Input: part model. Units: mm. Frame: model coordinates. Face numbers are marked on the shaded views. A direction names the side the tool comes from. Coordinates: 2 decimals unless noted, no trailing zeros. Write each loop counter-clockwise with the first axis right and the second up, starting at its lowest first coordinate (ties: lowest second). Pieces come first, ordered by that corner, then holes. Notation, with made-up numbers: (55.25, 3.25) - (70.25, 3.25) arc R20 cw to (70.25, 27.25) - close; hole circle Ø6 at (11, -13). An arc over 180 degrees is marked (long way). Put each result on its own line as item: value. Start each with the question number.
1. Cut plane B-B, the plane z = 0. Return loops of the section in (x, y).
2. Line query: line 1 (Y direction, x = -5.25, z = -2.5); line 2 (X direction, y = 45, z = 3.5); line 3 (X direction, y = 14, z = 2.5). Output: solid intervals per line, ascending.
3. Cut plane C-C, the plane y = 49.5. Return loops of the section in (x, z).
4. Cut plane D-D, the plane y = 9. Return loops of the section in (x, z), and give its area (3 significant figures).
5. Cut plane A-A, the plane x = 0. Return loops of the section in (y, z), and give its area (3 significant figures).
6. Access query for the marked faces 1, 2 and 3. Directions: +Z, -Z, +X, -X, +Y, -Y. A direction counts if a zero-diameter tool reaches every point of the face in a straight line with its end or side. Return the directions, or none.
7. Pin query (flat end, axial travel): pin 1 (4 mm diameter, centred on y = 76.5, z = 1.5, fed in from -X); pin 2 (3 mm diameter, centred on y = 67, z = 3, fed in from -X). Return the tip coordinate at first contact, or that it passes through.
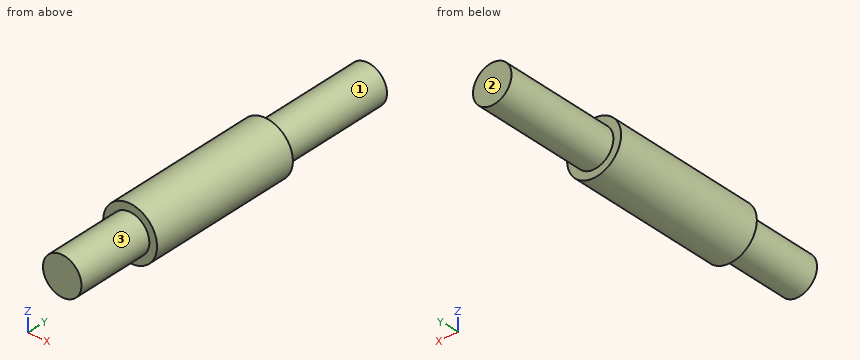
Autodesk Inventor part; units mm, degrees
ref_plane "YZ Plane" through (0, 0, 0) normal (1, 0, 0) x (0, 1, 0)
ref_plane "XZ Plane" through (0, 0, 0) normal (0, 1, 0) x (-1, 0, 0)
ref_plane "XY Plane" through (0, 0, 0) normal (0, 0, 1) x (1, 0, 0)
sketch "Sketch1" plane through (0, 0, 0) normal (0, 1, 0) x (-1, 0, 0)
  circle A0 centre (0, 0) radius 7
  dimension "d0" = 14
extrude "Extrusion1" add sketch "Sketch1" along normal blind 95
sketch "Sketch2" plane through (0, 0, 0) normal (0, -1, 0) x (1, 0, 0)
  circle A0 centre (0, 0) radius 7
  circle A1 centre (0, 0) radius 5
  dimension "d3" = 10
extrude "Extrusion2" cut sketch "Sketch2" against normal blind 20
sketch "Sketch3" plane through (0, 95, 0) normal (0, 1, 0) x (1, 0, 0)
  circle A0 centre (0, 0) radius 7
  circle A1 centre (0, 0) radius 5
  dimension "d6" = 14
  dimension "d7" = 10
extrude "Extrusion3" cut sketch "Sketch3" against normal blind 35
sketch "Sketch4" plane through (0, 95, 0) normal (0, 1, 0) x (1, 0, 0)
  circle A0 centre (0, 0) radius 5
  dimension "d10" = 10
extrude "Extrusion4" cut sketch "Sketch4" against normal blind 5
properties part number "trucj-10"
Report:
1. outline: (-7, 20) - (-5, 20) - (-5, 0) - (5, 0) - (5, 20) - (7, 20) - (7, 60) - (5, 60) - (5, 90) - (-5, 90) - (-5, 60) - (-7, 60) - close
2. line 1: y = 20 to 60
2. line 2: x = -6.06 to 6.06
2. line 3: x = -4.33 to 4.33
3. outline: circle Ø14 at (0, 0)
4. outline: circle Ø10 at (0, 0)
4. area: 78.5 mm^2
5. outline: (0, -5) - (20, -5) - (20, -7) - (60, -7) - (60, -5) - (90, -5) - (90, 5) - (60, 5) - (60, 7) - (20, 7) - (20, 5) - (0, 5) - close
5. area: 1,060 mm^2
6. face 1: +Y
6. face 2: +Z, -Z, +X, -X, +Y
6. face 3: -Y
7. pin 1: stops at x = -5
7. pin 2: stops at x = -4.77
